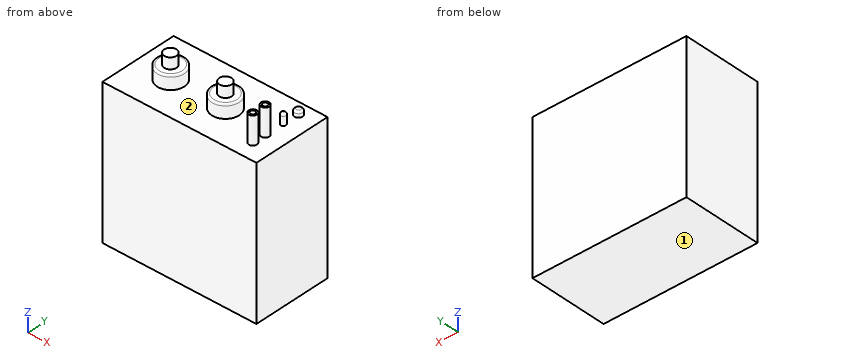
```python
from build123d import *

# Parameters (mm, degrees)
SKETCH1_W           = 142.875
SKETCH1_H           = 136.525
BOSS_EXTRUDE1_DEPTH = 73.025
SKETCH2_R           = 12.7
BOSS_EXTRUDE2_DEPTH = 12.7
FILLET2_SIZE        = 1.778
SKETCH3_R           = 5.715
BOSS_EXTRUDE3_DEPTH = 22.86
LPATTERN1_COUNT     = 2
LPATTERN1_PITCH     = 50.8
FILLET3_SIZE        = 1.778
SKETCH5_R           = 5.715
BOSS_EXTRUDE4_DEPTH = 10.16
SKETCH6_R           = 3.81
BOSS_EXTRUDE5_DEPTH = 5.08
FILLET4_SIZE        = 1.778
SKETCH7_R           = 2.5
BOSS_EXTRUDE6_DEPTH = 10.16
FILLET5_SIZE        = 2.032
SKETCH9_R           = 3.81
BOSS_EXTRUDE7_DEPTH = 25.4
SKETCH10_R          = 2.286
CUT_EXTRUDE1_DEPTH  = 25.4
LPATTERN2_COUNT     = 2
LPATTERN2_PITCH     = 12.7
SKETCH11_R          = 2.286
CUT_EXTRUDE2_DEPTH  = 25.4


with BuildPart() as part:
    # Sketch1 → Boss-Extrude1 (new body)
    with BuildSketch(Plane(origin=(0, 0, 0), x_dir=(1, 0, 0), z_dir=(0, 1, 0))):
        Rectangle(SKETCH1_W, SKETCH1_H)
    extrude(amount=BOSS_EXTRUDE1_DEPTH)

    # Sketch2 → Boss-Extrude2 (add)
    with BuildSketch(Plane.XY.offset(68.2625)):
        with Locations(Location((-38.516675306, 33.650171928, 0), (0, 0, 180))):
            Circle(SKETCH2_R)
    boss_extrude2 = extrude(amount=BOSS_EXTRUDE2_DEPTH)

    # Fillet2
    # a fillet whose section is not a circle: 1.778 mm, written as the material it takes off along each edge
    with BuildSketch(Plane(origin=(-38.516675306, 33.650171928, 80.9625), x_dir=(-1, 0, 0), z_dir=(0, 1, 0))) as fillet2_piece_1:
        with BuildLine():
            Bezier((12.7, -FILLET2_SIZE), (12.7, 0), (12.7 - FILLET2_SIZE, 0), weights=[1, 4.949747468, 1])
            Line((12.7 - FILLET2_SIZE, 0), (12.7, 0))
            Line((12.7, 0), (12.7, -FILLET2_SIZE))
        make_face()
    revolve(axis=Axis((-38.516675306, 33.650171928, 80.9625), (0, 0, 1)), mode=Mode.SUBTRACT)

    # Sketch3 → Boss-Extrude3 (add)
    with BuildSketch(Plane.XY.offset(68.2625)):
        with Locations((-38.516675306, 33.290572788)):
            Circle(SKETCH3_R)
    extrude(amount=BOSS_EXTRUDE3_DEPTH)

    # LPattern1: Boss-Extrude2 ×2
    with Locations(*[(i * LPATTERN1_PITCH, 0, 0) for i in range(1, LPATTERN1_COUNT)]):
        add(boss_extrude2)

    # Fillet3
    # a fillet whose section is not a circle: 1.778 mm, written as the material it takes off along each edge
    with BuildSketch(Plane(origin=(12.283324694, 33.650171928, 80.9625), x_dir=(-1, 0, 0), z_dir=(0, 1, 0))) as fillet3_piece_1:
        with BuildLine():
            Bezier((12.7, -FILLET3_SIZE), (12.7, 0), (12.7 - FILLET3_SIZE, 0), weights=[1, 4.949747468, 1])
            Line((12.7 - FILLET3_SIZE, 0), (12.7, 0))
            Line((12.7, 0), (12.7, -FILLET3_SIZE))
        make_face()
    revolve(axis=Axis((12.283324694, 33.650171928, 80.9625), (0, 0, 1)), mode=Mode.SUBTRACT)

    # Sketch5 → Boss-Extrude4 (add)
    with BuildSketch(Plane.XY.offset(80.9625)):
        with Locations((12.283324694, 33.650171928)):
            Circle(SKETCH5_R)
    extrude(amount=BOSS_EXTRUDE4_DEPTH)

    # Sketch6 → Boss-Extrude5 (add)
    with BuildSketch(Plane.XY.offset(68.2625)):
        with Locations(Location((54.627573576, 61.857843882, 0), (0, 0, 180))):
            Circle(SKETCH6_R)
    extrude(amount=BOSS_EXTRUDE5_DEPTH)

    # Fillet4
    # a fillet whose section is not a circle: 1.778 mm, written as the material it takes off along each edge
    with BuildSketch(Plane(origin=(54.627573576, 61.857843882, 73.3425), x_dir=(-1, 0, 0), z_dir=(0, 1, 0))) as fillet4_piece_1:
        with BuildLine():
            Bezier((3.81, -FILLET4_SIZE), (3.81, 0), (3.81 - FILLET4_SIZE, 0), weights=[1, 0.449977043, 1])
            Line((3.81 - FILLET4_SIZE, 0), (3.81, 0))
            Line((3.81, 0), (3.81, -FILLET4_SIZE))
        make_face()
    revolve(axis=Axis((54.627573576, 61.857843882, 73.3425), (0, 0, 1)), mode=Mode.SUBTRACT)

    # Sketch7 → Boss-Extrude6 (add)
    with BuildSketch(Plane.XY.offset(68.2625)):
        with Locations(Location((54.338250319, 46.619193899, 0), (0, 0, 180))):
            Circle(SKETCH7_R)
    extrude(amount=BOSS_EXTRUDE6_DEPTH)

    # Fillet5
    # a fillet whose section is not a circle: 2.032 mm, written as the material it takes off along each edge
    with BuildSketch(Plane(origin=(54.338250319, 46.619193899, 78.4225), x_dir=(-1, 0, 0), z_dir=(0, 1, 0))) as fillet5_piece_1:
        with BuildLine():
            Bezier((2.5, -FILLET5_SIZE), (2.5, 0), (2.5 - FILLET5_SIZE, 0), weights=[1, 0.565685425, 1])
            Line((2.5 - FILLET5_SIZE, 0), (2.5, 0))
            Line((2.5, 0), (2.5, -FILLET5_SIZE))
        make_face()
    revolve(axis=Axis((54.338250319, 46.619193899, 78.4225), (0, 0, 1)), mode=Mode.SUBTRACT)

    # Sketch9 → Boss-Extrude7 (add)
    with BuildSketch(Plane.XY.offset(68.2625)):
        with Locations(Location((53.431620425, 28.929804746, 0), (0, 0, 180))):
            Circle(SKETCH9_R)
    boss_extrude7 = extrude(amount=BOSS_EXTRUDE7_DEPTH)

    # Sketch10 → Cut-Extrude1 (cut)
    with BuildSketch(Plane.XY.offset(93.6625)):
        with Locations((53.431620425, 28.929804746)):
            Circle(SKETCH10_R)
    extrude(amount=-CUT_EXTRUDE1_DEPTH, mode=Mode.SUBTRACT)

    # LPattern2: Boss-Extrude7 ×2
    with Locations(*[(0, -i * LPATTERN2_PITCH, 0) for i in range(1, LPATTERN2_COUNT)]):
        add(boss_extrude7)

    # Sketch11 → Cut-Extrude2 (cut)
    with BuildSketch(Plane.XY.offset(93.6625)):
        with Locations((53.431620425, 16.229804746)):
            Circle(SKETCH11_R)
    extrude(amount=-CUT_EXTRUDE2_DEPTH, mode=Mode.SUBTRACT)


solid = part.part
```
CAD build for the part. Positions are in the model's coordinates, mm. Face numbers are marked on the shaded views. A direction names the side the tool comes from. Coordinates: 2 decimals unless noted, no trailing zeros. Order: outer loops, then holes, each group sorted by start corner. A loop starts at its lowest first (then second) coordinate and runs counter-clockwise, first axis right, second up. Notation, with made-up numbers: (15, 26) - (34, 26) arc R21 cw to (34, 49) - close; hole circle Ø4 at (41.5, 54). An arc over 180 degrees is marked (long way). Use a Markdown table: item, result. Add a question column.
(1) Which spindle directions (+Z, -Z, +X, -X, +Y, -Y) get a long thin tool onto all of the face, cutting with end or side? Do the marked faces 1 and 2. Say none if no direction does.
(2) Saw through at B-B (y = 7). Give the cut face in (x, z).
(3) Saw through at A-A (x = -54). Give the cut face in (y, z) (1 decimal), then the cut area to 3 significant figures.
(4) Flat gauge pins, fed straight in: pin 1 (0.5 mm diameter, centred on x = 54.5, y = 47, fed in from +Z); pin 2 (1.2 mm diameter, centred on x = 55, y = 61.5, fed in from +Z); pin 3 (3.5 mm diameter, centred on x = 13, y = 35, fed in from +Z). Where does each tip first touch, or does it go through?
(5) Drill centre lines: line 1 along Z through (x, y) = (50.5, 26); line 2 along X through (y, z) = (62, 71); line 3 along Z through (x, y) = (13, 44). Where is each one in solid material? Low to high. Write a range as [from, to].
Solved:
| question | item | result |
|---|---|---|
| 1 | face 1 | -Z, +X, -X, +Y, -Y |
| 1 | face 2 | +Z |
| 2 | outline | (-71.44, -68.26) - (71.44, -68.26) - (71.44, 68.26) - (-71.44, 68.26) - close |
| 3 | outline | (0, -68.3) - (73, -68.3) - (73, 68.3) - (0, 68.3) - close |
| 3 | area | 9,970 mm² |
| 4 | pin 1 | stops at z = 78.42 |
| 4 | pin 2 | stops at z = 73.34 |
| 4 | pin 3 | stops at z = 91.12 |
| 5 | line 1 | z = [-68.26, 68.26] |
| 5 | line 2 | x = [50.82, 58.43] |
| 5 | line 3 | z = [-68.26, 80.96] |
